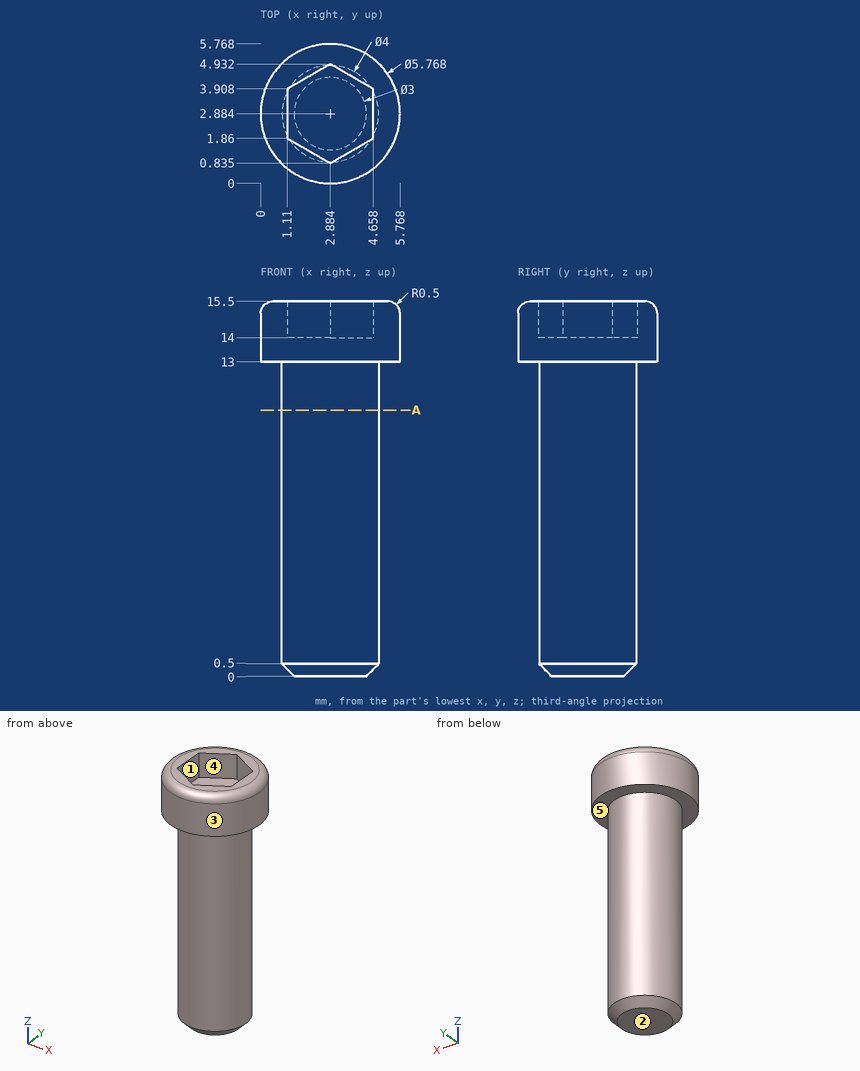
Source: three-view drawing plus pictorial views. Frame: mm from the lowest corner of the part. A direction names the side the tool comes from. Coordinates: 2 decimals unless noted, no trailing zeros. Order: outer loops, then holes, each group sorted by start corner. A loop starts at its lowest first (then second) coordinate and runs counter-clockwise, first axis right, second up.
1) First-contact query: P1, Ø2, axis at y = 3.5, z = 11, coming from the -X side; P2, Ø1.5, axis at x = 4.5, z = 5.5, coming from the +Y side; P3, Ø1.1, axis at x = 3.5, y = 3, coming from the +Z side. Flat tips, straight axial feed; report the tip coordinate or a pass-through.
Result sheet:
P1: stops at x = 0.88
P2: stops at y = 4.69
P3: stops at z = 14
2) Draft query along Y for the marked faces 1, 2 and 3. Return one class per face: released by +Y, released by -Y, zero draft, split by the parting line, or undercut.
Result sheet:
face 1: undercut
face 2: zero draft
face 3: split by the parting line
3) Set-up query: the marked faces 4 and 5. Return all of +Z, -Z, +X, -X, +Y, -Y with unobstructed straight access to the full face (end or side cutting, diameter ignored); none if empty.
Result sheet:
face 4: +Z
face 5: -Z
4) Section A-A (z = 11). Return loops of the section in (x, y), then the cut area to 3 significant figures.
Result sheet:
outline: circle Ø4 at (2.88, 2.88)
area: 12.6 mm2
5) Ray query, probe 1 along Z at (x, y) = (3.55, 3.1); probe 2 along Z at (x, y) = (0.5, 2.65); probe 3 along X at (y, z) = (2.85, 8.25). Return the intervals inside material, ascending.
Result sheet:
probe 1: z = 0 to 14
probe 2: z = 13 to 15.5
probe 3: x = 0.88 to 4.88
